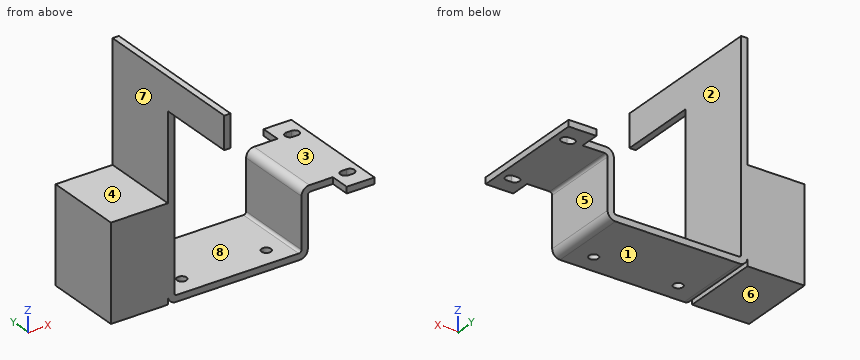
from build123d import *

# Parameters (mm, degrees)
F1_DEPTH  = 15
F2_W      = 2.4
F2_H      = 12.3
F3_DEPTH  = 30.5
F2_W_2    = 10.5
F2_H_2    = 2.4
F4_DEPTH  = 7.5
F5_W      = 10.5
F5_H      = 2.4
F6_DEPTH  = 7.5
F8_DEPTH  = 2.4
F9_R      = 3
F10_R     = 1
F11_W     = 30
F11_H     = 33
F11_H_2   = 3
F12_DEPTH = 21.6
F13_R     = 1.75
F14_DEPTH = 2.4


with BuildPart() as f1:
    # F0 (on Front) → F1 (new body, symmetric)
    with BuildSketch(Plane.XZ):
        Polygon((-53, 0), (0, 0), (0, 23), (20, 23), (20, 25.4), (-2.4, 25.4), (-2.4, 2.4), (-50.6, 2.4), (-50.6, 81), (-53, 81), align=None)
    extrude(amount=F1_DEPTH, both=True)

    # F2 (on face) → F3 (join)
    with BuildSketch(Plane.XZ.offset(15)):
        with Locations((-51.8, 74.85)):
            Rectangle(F2_W, F2_H)
    extrude(amount=F3_DEPTH)

    # F2 (on face) → F4 (join)
    with BuildSketch(Plane.XZ.offset(15)):
        with Locations((14.75, 24.2)):
            Rectangle(F2_W_2, F2_H_2)
    extrude(amount=F4_DEPTH)

    # F5 (on face) → F6 (join)
    with BuildSketch(Plane(origin=(0, 15, 0), x_dir=(-1, 0, 0), z_dir=(0, 1, 0))):
        with Locations((-14.75, 24.2)):
            Rectangle(F5_W, F5_H)
    extrude(amount=F6_DEPTH)

    # F7 (on face) → F8 (cut, through all)
    with BuildSketch(Plane.XY.offset(25.4)):
        with BuildLine():
            ThreePointArc((15.05, -13.499166898), (14.6169272275, -13.3134416807), (14.15, -13.25))
            ThreePointArc((14.15, -13.25), (12.4, -15), (14.15, -16.75))
            ThreePointArc((14.15, -16.75), (14.6169272275, -16.6865583193), (15.05, -16.500833102))
            ThreePointArc((15.05, -16.500833102), (14.2, -15), (15.05, -13.499166898))
        make_face()
        with BuildLine():
            ThreePointArc((15.9, -15), (15.6727442333, -14.1375905845), (15.05, -13.499166898))
            ThreePointArc((15.05, -13.499166898), (14.2, -15), (15.05, -16.500833102))
            ThreePointArc((15.05, -16.500833102), (15.6727442333, -15.8624094155), (15.9, -15))
        make_face()
        with BuildLine():
            ThreePointArc((15.95, -13.25), (15.4830727725, -13.3134416807), (15.05, -13.499166898))
            ThreePointArc((15.05, -13.499166898), (15.6727442333, -14.1375905845), (15.9, -15))
            ThreePointArc((15.9, -15), (15.6727442333, -15.8624094155), (15.05, -16.500833102))
            ThreePointArc((15.05, -16.500833102), (15.4830727725, -16.6865583193), (15.95, -16.75))
            ThreePointArc((15.95, -16.75), (17.1874368671, -16.2374368671), (17.7, -15))
            ThreePointArc((17.7, -15), (17.1874368671, -13.7625631329), (15.95, -13.25))
        make_face()
        with BuildLine():
            Line((15.95, -13.25), (14.15, -13.25))
            ThreePointArc((14.15, -13.25), (14.6169272275, -13.3134416807), (15.05, -13.499166898))
            ThreePointArc((15.05, -13.499166898), (15.4830727725, -13.3134416807), (15.95, -13.25))
        make_face()
        with BuildLine():
            ThreePointArc((15.05, -16.500833102), (14.6169272275, -16.6865583193), (14.15, -16.75))
            Line((14.15, -16.75), (15.95, -16.75))
            ThreePointArc((15.95, -16.75), (15.4830727725, -16.6865583193), (15.05, -16.500833102))
        make_face()
        with BuildLine():
            ThreePointArc((15.05, 16.500833102), (14.6169272275, 16.6865583193), (14.15, 16.75))
            ThreePointArc((14.15, 16.75), (12.4, 15), (14.15, 13.25))
            ThreePointArc((14.15, 13.25), (14.6169272275, 13.3134416807), (15.05, 13.499166898))
            ThreePointArc((15.05, 13.499166898), (14.2, 15), (15.05, 16.500833102))
        make_face()
        with BuildLine():
            ThreePointArc((15.9, 15), (15.6727442333, 15.8624094155), (15.05, 16.500833102))
            ThreePointArc((15.05, 16.500833102), (14.2, 15), (15.05, 13.499166898))
            ThreePointArc((15.05, 13.499166898), (15.6727442333, 14.1375905845), (15.9, 15))
        make_face()
        with BuildLine():
            ThreePointArc((15.95, 16.75), (15.4830727725, 16.6865583193), (15.05, 16.500833102))
            ThreePointArc((15.05, 16.500833102), (15.6727442333, 15.8624094155), (15.9, 15))
            ThreePointArc((15.9, 15), (15.6727442333, 14.1375905845), (15.05, 13.499166898))
            ThreePointArc((15.05, 13.499166898), (15.4830727725, 13.3134416807), (15.95, 13.25))
            ThreePointArc((15.95, 13.25), (17.1874368671, 13.7625631329), (17.7, 15))
            ThreePointArc((17.7, 15), (17.1874368671, 16.2374368671), (15.95, 16.75))
        make_face()
        with BuildLine():
            Line((15.95, 16.75), (14.15, 16.75))
            ThreePointArc((14.15, 16.75), (14.6169272275, 16.6865583193), (15.05, 16.500833102))
            ThreePointArc((15.05, 16.500833102), (15.4830727725, 16.6865583193), (15.95, 16.75))
        make_face()
        with BuildLine():
            ThreePointArc((15.05, 13.499166898), (14.6169272275, 13.3134416807), (14.15, 13.25))
            Line((14.15, 13.25), (15.95, 13.25))
            ThreePointArc((15.95, 13.25), (15.4830727725, 13.3134416807), (15.05, 13.499166898))
        make_face()
    extrude(amount=-F8_DEPTH, mode=Mode.SUBTRACT)

    # F9
    f9_edges = [f1.edges().sort_by_distance(p)[0] for p in [
        (-2.4, 0, 25.4),
        (0, 0, 0),
        (-53, 0, 0),
    ]]
    fillet(f9_edges, radius=F9_R)

    # F10
    f10_edges = [f1.edges().sort_by_distance(p)[0] for p in [
        (-50.6, 0, 2.4),
        (-2.4, 0, 2.4),
        (0, 0, 23),
    ]]
    fillet(f10_edges, radius=F10_R)

    # F11 (on face) → F12 (join)
    with BuildSketch(Plane(origin=(-53, 0, 0), x_dir=(0, -1, 0), z_dir=(-1, 0, 0))):
        with Locations((0, 19.5)):
            Rectangle(F11_W, F11_H)
        with Locations((0, 1.5)):
            Rectangle(F11_W, F11_H_2)
    extrude(amount=F12_DEPTH)

    # F13 (on face) → F14 (cut, through all)
    with BuildSketch(Plane(origin=(0, 0, 0), x_dir=(1, 0, 0), z_dir=(0, 0, -1))):
        with Locations((-42.5, 7.5)):
            Circle(F13_R)
        with Locations((-10.5, 7.5)):
            Circle(F13_R)
    extrude(amount=-F14_DEPTH, mode=Mode.SUBTRACT)


solid = f1.part
Could you check a few things on this model? Use its own coordinates, in mm. Face numbers are marked on the shaded views. A direction names the side the tool comes from. Give positions to 0.01 mm unless a question says otherwise; leave off trailing zeros. Write each loop counter-clockwise with the first axis right and the second up, starting at its lowest first coordinate (ties: lowest second). Pieces come first, ordered by that corner, then holes. Notation, with made-up numbers: (70, 47.5) -> (114, 47.5) arc R28 ccw to (114, 73.5) -> close; hole circle Ø1 at (76.25, 55). An arc over 180 degrees is marked (long way). Answer as CSV lines item,"result". Start each with the question number.
(1) I'm going to push flat-ended pins straight in: pin 1 Ø2.5 at (y, z) = (-19.5, 24.5) entering from -X; pin 2 Ø0.7 at (x, z) = (16.5, 23.5) entering from -Y; pin 3 Ø6.5 at (x, y) = (-65, -1) entering from +Z; pin 4 Ø15 at (y, z) = (1.5, 16) entering from +X. Where does each tip first touch, or does it pass through?
(2) If we section it at B-B, the plane y = 12: Write out the boundary of the cut face in (x, z), and give its area (3 significant figures).
(3) If we section it at C-C, the plane y = -7.5: Write out the boundary of the cut face in (x, z), and give its area (3 significant figures).
(4) If we section it at A-A, the plane x = -42.5: Write out the boundary of the cut face in (y, z).
(5) Please list where these lines run through material, in increasing order: line 1 (Y direction, x = -10.5, z = 1.7); line 2 (X direction, y = -10, z = 21); line 3 (X direction, y = -7.5, z = 1).
(6) Which directions (+Z, -Z, +X, -X, +Y, -Y) give clear straight access to the entire face, cutting with the end or side of a thin tool? Please do the marked faces 1, 2, 3, 4 and 5.
(7) If we mould it in two halves opening along X, with no side actions, what happens to the marked faces 6, 7 and 8? For each: +X half, -X half, draft (parallel to the pull), parting line (faces both ways), or undercut.
(8) If we section it at D-D, the plane z = 33: Write out the boundary of the cut face in (x, y), and give its area (3 significant figures).
Answer list:
1,pin 1,"x = 9.5"
1,pin 2,"y = -22.5"
1,pin 3,"z = 36"
1,pin 4,"x = 20"
2,outline,"(-74.6, 0) -> (-53, 0) -> (-53, 3) arc R3 ccw to (-50, 0) -> (-3, 0) arc R3 ccw to (0, 3) -> (0, 22) arc R1 cw to (1, 23) -> (20, 23) -> (20, 25.4) -> (0.6, 25.4) arc R3 ccw to (-2.4, 22.4) -> (-2.4, 3.4) arc R1 cw to (-3.4, 2.4) -> (-49.6, 2.4) arc R1 cw to (-50.6, 3.4) -> (-50.6, 81) -> (-53, 81) -> (-53, 36) -> (-74.6, 36) -> close"
2,area,"1,190 mm^2"
3,outline,"(-74.6, 0) -> (-53, 0) -> (-53, 3) arc R3 ccw to (-50, 0) -> (-44.25, 0) -> (-44.25, 2.4) -> (-49.6, 2.4) arc R1 cw to (-50.6, 3.4) -> (-50.6, 81) -> (-53, 81) -> (-53, 36) -> (-74.6, 36) -> close; (-40.75, 0) -> (-12.25, 0) -> (-12.25, 2.4) -> (-40.75, 2.4) -> close; (-8.75, 0) -> (-3, 0) arc R3 ccw to (0, 3) -> (0, 22) arc R1 cw to (1, 23) -> (20, 23) -> (20, 25.4) -> (0.6, 25.4) arc R3 ccw to (-2.4, 22.4) -> (-2.4, 3.4) arc R1 cw to (-3.4, 2.4) -> (-8.75, 2.4) -> close"
3,area,"1,170 mm^2"
4,outline,"(-15, 0) -> (-9.25, 0) -> (-9.25, 2.4) -> (-15, 2.4) -> close; (-5.75, 0) -> (15, 0) -> (15, 2.4) -> (-5.75, 2.4) -> close"
5,line 1,"-15 to -9.25, -5.75 to 15"
5,line 2,"-74.6 to -50.6, -2.4 to 0"
5,line 3,"-74.6 to -53, -52.24 to -44.25, -40.75 to -12.25, -8.75 to -0.76"
6,face 1,"-Z, +X, -X, +Y, -Y"
6,face 2,"+Z, +Y, -Y"
6,face 3,"+Z, +X, +Y, -Y"
6,face 4,"+Z, -X, +Y, -Y"
6,face 5,"-Z, +X, +Y, -Y"
7,face 6,"draft"
7,face 7,"-X half"
7,face 8,"undercut"
8,outline,"(-74.6, -15) -> (-50.6, -15) -> (-50.6, 15) -> (-74.6, 15) -> close"
8,area,"720 mm^2"
